Autodesk Inventor part; units mm, degrees
ref_plane "YZ Plane" through (0, 0, 0) normal (1, 0, 0) x (0, 1, 0)
ref_plane "XZ Plane" through (0, 0, 0) normal (0, 1, 0) x (-1, 0, 0)
ref_plane "XY Plane" through (0, 0, 0) normal (0, 0, 1) x (1, 0, 0)
sketch "Esboço1" plane through (0, 0, 0) normal (0, 1, 0) x (-1, 0, 0)
  arc A0 (-491.7313, -306.4749) -> (358.2687, 543.5251) centre (-491.7313, 543.5251) ccw
  arc A1 (-491.7313, -346.4749) -> (398.2687, 543.5251) centre (-491.7313, 543.5251) ccw
  line L0 (358.2687, 543.5251) -> (398.2687, 543.5251)
  line L1 (-491.7313, -306.4749) -> (-491.7313, -346.4749)
  point P0 (0, 0)
  dimension "d0" = 850
  dimension "d1" = 890
extrude "Extrusão1" add sketch "Esboço1" along normal blind 3
sketch "Esboço2" plane through (0, 3, 0) normal (0, 1, 0) x (1, 0, 0)
  circle A0 centre (-378.2687, -536.0251) radius 2.5
  circle A1 centre (484.2313, 326.4749) radius 2.5
  line L0 (491.7313, 306.4749) -> (491.7313, 346.4749)
  line L1 (-398.2687, -543.5251) -> (-358.2687, -543.5251)
  point P0 (0, 0)
  dimension "d16" = 5
  dimension "d17" = 5
  dimension "d18" = 7.5
  dimension "d19" = 20
  dimension "d20" = 7.5
  dimension "d21" = 20
hole "Furo1" at (-378.2687, 3, 536.0251) at (484.2313, 3, -326.4749) direction (0, -1, 0) diameter 5 end through all
properties part number "Arco médio" material "Alumínio 6061"
Part model, mm, in its own coordinate system. Round coordinates to 2 decimals unless told otherwise and drop trailing zeros. Loops run counter-clockwise (first coordinate to the right, second up) from the corner with the lowest first, then second, coordinate; pieces in that order, holes last.
Item 1: Cut at A-A, the plane y = 1.85. Give the cut face in (x, z).
Item 2: Cut at B-B, the plane x = -132. Give the cut face in (y, z), then the cut area to 3 significant figures.
Item 3: Drill centre lines: line 1 (Z direction, x = -111, y = 2); line 2 (Z direction, x = 155.5, y = 1.95); line 3 (X direction, y = 0.95, z = -67). Where is each one in solid material? Low to high.
Item 4: Cut at C-C, the plane z = -212. Give the cut face in (x, y).
Item 5: Drop flat-ended pins along their axis: P1, Ø1, axis at y = 1, z = 227, coming from the -X side; P2, Ø4.5, axis at x = -378.27, z = 536.03, coming from the +Y side. Give the stop position or say it passes through.
A:
1. outline: (-398.27, 543.53) arc R890 ccw to (491.73, -346.47) - (491.73, -306.47) arc R850 cw to (-358.27, 543.53) - close; hole circle Ø5 at (-378.27, 536.03); hole circle Ø5 at (484.23, -326.47)
2. outline: (0, -91.34) - (3, -91.34) - (3, -33.93) - (0, -33.93) - close
2. area: 172 mm2
3. line 1: z = -111.31 to -55.82
3. line 2: z = -280.52 to -237.15
3. line 3: x = -155.85 to -99.67
4. outline: (21.33, 0) - (102.27, 0) - (102.27, 3) - (21.33, 3) - close
5. P1: stops at x = -340.27
5. P2: passes through
